```python
from build123d import *

# Parameters (mm, degrees)
SKETCH1_R           = 5.45
BOSS_EXTRUDE1_DEPTH = 50
SKETCH6_R           = 2.5
BOSS_EXTRUDE2_DEPTH = 2.5
SKETCH7_R           = 2.65
CUT_EXTRUDE1_DEPTH  = 3
JOIN1_DEPTH         = 5


# Read off the part's stored shape, not the designer's step: Join1
with BuildPart() as part:
    # Sketch1 → Boss-Extrude1 (new body)
    with BuildSketch(Plane.XY):
        Circle(SKETCH1_R)
    extrude(amount=BOSS_EXTRUDE1_DEPTH)

    # Sketch6 → Boss-Extrude2 (add)
    with BuildSketch(Plane(origin=(0, 0, 0), x_dir=(-1, 0, 0), z_dir=(0, 0, -1))):
        Circle(SKETCH6_R)
    extrude(amount=BOSS_EXTRUDE2_DEPTH)

    # Sketch7 → Cut-Extrude1 (cut)
    with BuildSketch(Plane.XY.offset(50)):
        Circle(SKETCH7_R)
    extrude(amount=-CUT_EXTRUDE1_DEPTH, mode=Mode.SUBTRACT)

    # Join1 outline → Join1 (add)
    with BuildSketch(Plane.XY):
        with BuildLine():
            ThreePointArc((3.905791733, -7.336608426), (5.093273997, -9.101255459), (6.993020796, -10.05784073))
            ThreePointArc((6.993020796, -10.05784073), (7.262719681, -9.864856959), (7.527095748, -9.664643274))
            ThreePointArc((7.527095748, -9.664643274), (7.177895055, -7.56651264), (5.845552604, -5.908514788))
            ThreePointArc((5.845552604, -5.908514788), (6.492103401, -5.189761622), (7.050819075, -4.400793408))
            ThreePointArc((7.050819075, -4.400793408), (8.961532399, -5.335281436), (11.085054023, -5.213835182))
            ThreePointArc((11.085054023, -5.213835182), (11.222128224, -4.911856891), (11.350977771, -4.60627872))
            ThreePointArc((11.350977771, -4.60627872), (9.999495783, -2.963844637), (8.016654448, -2.194147603))
            ThreePointArc((8.016654448, -2.194147603), (8.21720728, -1.248413703), (8.306585141, -0.28578935))
            ThreePointArc((8.306585141, -0.28578935), (10.428555432, -0.13972306), (12.206855977, 1.027213293))
            ThreePointArc((12.206855977, 1.027213293), (12.174576572, 1.357271264), (12.133374467, 1.686334497))
            ThreePointArc((12.133374467, 1.686334497), (10.141739691, 2.432983143), (8.039700207, 2.10813966))
            ThreePointArc((8.039700207, 2.10813966), (7.740517104, 3.027445658), (7.336608426, 3.905791733))
            ThreePointArc((7.336608426, 3.905791733), (9.101255459, 5.093273997), (10.05784073, 6.993020796))
            ThreePointArc((10.05784073, 6.993020796), (9.864856959, 7.262719681), (9.664643274, 7.527095748))
            ThreePointArc((9.664643274, 7.527095748), (7.56651264, 7.177895055), (5.908514788, 5.845552604))
            ThreePointArc((5.908514788, 5.845552604), (5.189761622, 6.492103401), (4.400793408, 7.050819075))
            ThreePointArc((4.400793408, 7.050819075), (5.335281436, 8.961532399), (5.213835182, 11.085054023))
            ThreePointArc((5.213835182, 11.085054023), (4.911856891, 11.222128224), (4.60627872, 11.350977771))
            ThreePointArc((4.60627872, 11.350977771), (2.963844637, 9.999495783), (2.194147603, 8.016654448))
            ThreePointArc((2.194147603, 8.016654448), (1.248413703, 8.21720728), (0.28578935, 8.306585141))
            ThreePointArc((0.28578935, 8.306585141), (0.13972306, 10.428555432), (-1.027213293, 12.206855977))
            ThreePointArc((-1.027213293, 12.206855977), (-1.357271264, 12.174576572), (-1.686334497, 12.133374467))
            ThreePointArc((-1.686334497, 12.133374467), (-2.432983143, 10.141739691), (-2.10813966, 8.039700207))
            ThreePointArc((-2.10813966, 8.039700207), (-3.027445658, 7.740517104), (-3.905791733, 7.336608426))
            ThreePointArc((-3.905791733, 7.336608426), (-5.093273997, 9.101255459), (-6.993020796, 10.05784073))
            ThreePointArc((-6.993020796, 10.05784073), (-7.262719681, 9.864856959), (-7.527095748, 9.664643274))
            ThreePointArc((-7.527095748, 9.664643274), (-7.177895055, 7.56651264), (-5.845552604, 5.908514788))
            ThreePointArc((-5.845552604, 5.908514788), (-6.492103401, 5.189761622), (-7.050819075, 4.400793408))
            ThreePointArc((-7.050819075, 4.400793408), (-8.961532399, 5.335281436), (-11.085054023, 5.213835182))
            ThreePointArc((-11.085054023, 5.213835182), (-11.222128224, 4.911856891), (-11.350977771, 4.60627872))
            ThreePointArc((-11.350977771, 4.60627872), (-9.999495783, 2.963844637), (-8.016654448, 2.194147603))
            ThreePointArc((-8.016654448, 2.194147603), (-8.21720728, 1.248413703), (-8.306585141, 0.28578935))
            ThreePointArc((-8.306585141, 0.28578935), (-10.428555432, 0.13972306), (-12.206855977, -1.027213293))
            ThreePointArc((-12.206855977, -1.027213293), (-12.174576572, -1.357271264), (-12.133374467, -1.686334497))
            ThreePointArc((-12.133374467, -1.686334497), (-10.141739691, -2.432983143), (-8.039700207, -2.10813966))
            ThreePointArc((-8.039700207, -2.10813966), (-7.740517104, -3.027445658), (-7.336608426, -3.905791733))
            ThreePointArc((-7.336608426, -3.905791733), (-9.101255459, -5.093273997), (-10.05784073, -6.993020796))
            ThreePointArc((-10.05784073, -6.993020796), (-9.864856959, -7.262719681), (-9.664643274, -7.527095748))
            ThreePointArc((-9.664643274, -7.527095748), (-7.56651264, -7.177895055), (-5.908514788, -5.845552604))
            ThreePointArc((-5.908514788, -5.845552604), (-5.189761622, -6.492103401), (-4.400793408, -7.050819075))
            ThreePointArc((-4.400793408, -7.050819075), (-5.335281436, -8.961532399), (-5.213835182, -11.085054023))
            ThreePointArc((-5.213835182, -11.085054023), (-4.911856891, -11.222128224), (-4.60627872, -11.350977771))
            ThreePointArc((-4.60627872, -11.350977771), (-2.963844637, -9.999495783), (-2.194147603, -8.016654448))
            ThreePointArc((-2.194147603, -8.016654448), (-1.248413703, -8.21720728), (-0.28578935, -8.306585141))
            ThreePointArc((-0.28578935, -8.306585141), (-0.13972306, -10.428555432), (1.027213293, -12.206855977))
            ThreePointArc((1.027213293, -12.206855977), (1.357271264, -12.174576572), (1.686334497, -12.133374467))
            ThreePointArc((1.686334497, -12.133374467), (2.432983143, -10.141739691), (2.10813966, -8.039700207))
            ThreePointArc((2.10813966, -8.039700207), (3.027445658, -7.740517104), (3.905791733, -7.336608426))
        make_face()
    extrude(amount=JOIN1_DEPTH)


solid = part.part
```
For this review, take the finished solid that the model builds, in its own axes (mm). Round coordinates to 2 decimals unless told otherwise and drop trailing zeros. Write each loop counter-clockwise with the first axis right and the second up, starting at its lowest first coordinate (ties: lowest second). Pieces come first, ordered by that corner, then holes. Notation, with made-up numbers: M 27.25,73 L 77.25,73 A13 ccw 77.25,96 Z; hole C -29,21 d2. An arc over 180 degrees is marked long. One line per item, written item: value. Start each with the question number.
(1) Insertion check: pin 1 (10 mm diameter, centred on y = 9, z = 30.5, fed in from +X); pin 2 (6 mm diameter, centred on y = 3, z = 13, fed in from -X); pin 3 (3 mm diameter, centred on x = 4, y = -2.5, fed in from -Z); pin 4 (5 mm diameter, centred on y = 8, z = 17.5, fed in from -X). Each pin has a flat end and moves straight along its axis. Give the tip position at first contact, or say it passes through.
(2) We need section A-A (z = 10). Give the boundary of the cut face in (x, y), and give its area (3 significant figures).
(3) The part is to be moulded in two halves that separate along Y. For faces 1 (the flat face through (1.8, -5.4, 5)), 2 (the cylindrical face through (0.54, -2.44, -1.23)), 3 (the cylindrical face through (10.17, 2.43, 2.46)), 4 (the cylindrical face through (-3.015, 7.745, 2.465)), say which applies: released by +Y, released by -Y, zero draft, split by the parting line, or undercut.
(4) Wall thickness on line 1 (Y direction, x = 0, z = 48.2); line 2 (Z direction, x = -1, y = 0.5); line 3 (Z direction, x = 8.75, y = -4.25): over which ranges is each line inside the solid? List them lowest first.
Result:
1. pin 1: x = 3.7
1. pin 2: x = -5.45
1. pin 3: z = 0
1. pin 4: through
2. outline: C 0,0 d10.9
2. area: 93.3 mm²
3. face 1: zero draft
3. face 2: split by the parting line
3. face 3: undercut
3. face 4: undercut
4. line 1: -5.45 to -2.65, 2.65 to 5.45
4. line 2: -2.5 to 47
4. line 3: 0 to 5
